```python
from build123d import *

# Parameters (mm, degrees)
SKETCH_1_R               = 29.5
EXTRUDE_1_DEPTH          = 11
SKETCH_2_R               = 15
EXTRUDE_2_DEPTH          = 33
SKETCH_3_W               = 12.5
SKETCH_3_H               = 12.5
EXTRUDE_3_DEPTH          = 12
SKETCH_4_R               = 2.75
CUT_EXTRUDE_1_DEPTH      = 12
PATTERN_CIRCULAR_1_COUNT = 4
SKETCH_5_R               = 1.5
CUT_EXTRUDE_2_DEPTH      = 10


with BuildPart() as part:
    # 草图1 → 凸台-拉伸1 (new body)
    with BuildSketch(Plane(origin=(0, 0, 0), x_dir=(1, 0, 0), z_dir=(0, 1, 0))):
        Circle(SKETCH_1_R)
    extrude(amount=EXTRUDE_1_DEPTH)

    # 草图2 → 凸台-拉伸2 (add)
    with BuildSketch(Plane(origin=(0, 11, 0), x_dir=(1, 0, 0), z_dir=(0, 1, 0))):
        Circle(SKETCH_2_R)
    extrude(amount=EXTRUDE_2_DEPTH)

    # 草图3 → 凸台-拉伸3 (add)
    with BuildSketch(Plane(origin=(0, 44, 0), x_dir=(1, 0, 0), z_dir=(0, 1, 0))):
        Rectangle(SKETCH_3_W, SKETCH_3_H)
    extrude(amount=EXTRUDE_3_DEPTH)

    # 草图4 → 切除-拉伸1 (cut)
    with BuildSketch(Plane(origin=(0, 11, 0), x_dir=(1, 0, 0), z_dir=(0, 1, 0))):
        with Locations((16.086679272, 16.086679272)):
            Circle(SKETCH_4_R)
    cut_extrude_1 = extrude(amount=-CUT_EXTRUDE_1_DEPTH, mode=Mode.SUBTRACT)

    # 阵列(圆周)1: 切除-拉伸1 ×4 about axis
    pattern_circular_1_axis = Axis((0, 0, 0), (0, 1, 0))
    for i in range(1, PATTERN_CIRCULAR_1_COUNT):
        add(cut_extrude_1.rotate(pattern_circular_1_axis, i * 360 / PATTERN_CIRCULAR_1_COUNT), mode=Mode.SUBTRACT)

    # 草图5 → 切除-拉伸2 (cut)
    with BuildSketch(Plane(origin=(0, 56, 0), x_dir=(1, 0, 0), z_dir=(0, 1, 0))):
        Circle(SKETCH_5_R)
    extrude(amount=-CUT_EXTRUDE_2_DEPTH, mode=Mode.SUBTRACT)


solid = part.part
```
Read the model definition and answer for the solid it produces. Units are mm, in the model's axes. A direction names the side the tool comes from. Give positions to 0.01 mm unless a question says otherwise; leave off trailing zeros. Loops run counter-clockwise (first coordinate to the right, second up) from the corner with the lowest first, then second, coordinate; pieces in that order, holes last.
Item 1: The part is cut by section C-C (y = 7). Write down the section's boundary in (x, z).
Item 2: The part is cut by section A-A (x = 0). Write down the section's boundary in (y, z).
Item 3: Each of these flat-tipped pins is pushed along its axis until it touches: pin 1 Ø12 at (y, z) = (10.5, -23.5) entering from +X; pin 2 Ø3.5 at (y, z) = (47.5, -1) entering from +X; pin 3 Ø10 at (y, z) = (14.5, -3) entering from +X; pin 4 Ø4 at (x, z) = (-8.5, -0.5) entering from +Y. Where does it stop, or does it pass through?
Item 4: For faces 1 (the flat face through (0, 50, -6.25)), 2 (the flat face through (-6.25, 50, 0)), 3 (the flat face through (6.25, 50, 0)), determine the directions among +Z, -Z, +X, -X, +Y, -Y from which every point of the face is accessible in a straight line to the end or side of a thin tool.
Item 5: The part is cut by section B-B (z = 0). Write down the section's boundary in (x, y), and give its area (3 significant figures).
Item 6: The mould has two halves that part along Z. Classify faces 4 (the cylindrical face through (-18.813, 5.577, -15.729)), 5 (the cylindrical face through (-14.985, 27.269, -0.66)), 6 (the flat face through (0, 50, 6.25)): released by +Z, released by -Z, zero draft, split by the parting line, or undercut.
Item 7: The part is cut by section D-D (z = -17.5). Write down the section's boundary in (x, y).
Item 8: Find the intervals of material crossed by line 1 along Z through (x, y) = (0, 50); line 2 along Z through (x, y) = (17.5, 9), in increasing order.
Taken from the geometry:
1. outline: circle Ø59 at (0, 0); hole circle Ø5.5 at (-16.09, -16.09); hole circle Ø5.5 at (-16.09, 16.09); hole circle Ø5.5 at (16.09, -16.09); hole circle Ø5.5 at (16.09, 16.09)
2. outline: (0, -29.5) - (11, -29.5) - (11, -15) - (44, -15) - (44, -6.25) - (56, -6.25) - (56, -1.5) - (46, -1.5) - (46, 1.5) - (56, 1.5) - (56, 6.25) - (44, 6.25) - (44, 15) - (11, 15) - (11, 29.5) - (0, 29.5) - close
3. pin 1: stops at x = 23.75
3. pin 2: stops at x = 6.25
3. pin 3: stops at x = 29.5
3. pin 4: stops at y = 44
4. face 1: -Z, +X, -X, +Y
4. face 2: +Z, -Z, -X, +Y
4. face 3: +Z, -Z, +X, +Y
5. outline: (-29.5, 0) - (29.5, 0) - (29.5, 11) - (15, 11) - (15, 44) - (6.25, 44) - (6.25, 56) - (1.5, 56) - (1.5, 46) - (-1.5, 46) - (-1.5, 56) - (-6.25, 56) - (-6.25, 44) - (-15, 44) - (-15, 11) - (-29.5, 11) - close
5. area: 1,760 mm2
6. face 4: undercut
6. face 5: split by the parting line
6. face 6: released by +Z
7. outline: (-23.75, 0) - (-18.45, 0) - (-18.45, 11) - (-23.75, 11) - close; (-13.73, 0) - (13.73, 0) - (13.73, 11) - (-13.73, 11) - close; (18.45, 0) - (23.75, 0) - (23.75, 11) - (18.45, 11) - close
8. line 1: z = -6.25 to -1.5, 1.5 to 6.25
8. line 2: z = -23.75 to -18.45, -13.73 to 13.73, 18.45 to 23.75
